Verification items for the finished model (mm, model axes). Give positions to 0.01 mm unless a question says otherwise; leave off trailing zeros. Write each loop counter-clockwise with the first axis right and the second up, starting at its lowest first coordinate (ties: lowest second). Pieces come first, ordered by that corner, then holes. Notation, with made-up numbers: (-20.75, -20.5) -> (-14.75, -20.5) arc R25 cw to (-14.75, -8.5) -> close; hole circle Ø9 at (-6.5, 77.25). An arc over 180 degrees is marked (long way). Answer as CSV lines item,"result". Start each with the question number.
1) Sectioned sample at A-A on x = 0. Record the cut outline in (y, z), and give its area (3 significant figures).
2) Sectioned sample at D-D on y = -49.5. Record the cut outline in (x, z), and give its area (3 significant figures).
3) Mould release check, pull along X, two halves, no side actions. Record for faces 1 (the flat face through (5.38, -27.3, 2.96)), 2 (the cylindrical face through (11.175, -20.583, 2.958)), 3 (the flat face through (16, -20, 6)): released by +X, released by -X, zero draft, split by the parting line, or undercut.
4) Gauge pin test, flat end, axial feed: pin 1 Ø3 at (x, y) = (9.7, -19.97) entering from +Z. Record the tip position at first contact, or that the pin passes through.
5) Material ranges on L1, parallel to Y at x = 0, z = 3.85; L2, parallel to Y at x = 11, z = 2.45; L3, parallel to X at y = -19, z = 4.7, recorded low to high.
6) Sectioned sample at B-B on y = 0. Record the cut outline in (x, z).
7) Sectioned sample at C-C on z = 0.9. Record the cut outline in (x, y), and give its area (3 significant figures).
```python
from build123d import *

# Parameters (mm, degrees)
SKETCH1_R           = 1.6
BOSS_EXTRUDE1_DEPTH = 6


with BuildPart() as part:
    # Sketch1 → Boss-Extrude1 (new body)
    with BuildSketch(Plane.XY):
        Polygon((-20.528429637, 7.707371577), (6.638285905, 20.898640153), (46.575535608, -61.35), (30.575535608, -61.35), align=None)
        Circle(SKETCH1_R, mode=Mode.SUBTRACT)
        with Locations((9.696892794, -19.970234604)):
            Circle(SKETCH1_R, mode=Mode.SUBTRACT)
    extrude(amount=BOSS_EXTRUDE1_DEPTH)


solid = part.part
```
Ans:
1,outline,"(-20.03, 0) -> (-1.6, 0) -> (-1.6, 6) -> (-20.03, 6) -> close; (1.6, 0) -> (17.68, 0) -> (17.68, 6) -> (1.6, 6) -> close"
1,area,"207 mm²"
2,outline,"(21.81, 0) -> (40.82, 0) -> (40.82, 6) -> (21.81, 6) -> close"
2,area,"114 mm²"
3,face 1,"released by -X"
3,face 2,"undercut"
3,face 3,"zero draft"
4,pin 1,"passes through"
5,L1,"y = -20.03 to -1.6, 1.6 to 17.68"
5,L2,"y = -34.9 to -20.9, -19.04 to 11.92"
5,L3,"x = -0.76 to 8.42, 10.97 to 26.01"
6,outline,"(-14.82, 0) -> (-1.6, 0) -> (-1.6, 6) -> (-14.82, 6) -> close; (1.6, 0) -> (16.79, 0) -> (16.79, 6) -> (1.6, 6) -> close"
7,outline,"(-20.53, 7.71) -> (30.58, -61.35) -> (46.58, -61.35) -> (6.64, 20.9) -> close; hole circle Ø3.2 at (0, 0); hole circle Ø3.2 at (9.7, -19.97)"
7,area,"1,920 mm²"
